Autodesk Inventor part; units mm, degrees
ref_plane "XZ Plane" through (0, 0, 0) normal (0, 1, 0) x (-1, 0, 0)
ref_plane "XY Plane" through (0, 0, 0) normal (0, 0, 1) x (1, 0, 0)
sketch "Sketch1" plane through (0, 0, 0) normal (1, 0, 0) x (0, 1, 0)
  line L0 (0, 67.4997) -> (0, -67.4997)
  line L1 (0, 60) -> (8, 60)
  line L2 (8, 60) -> (8, 42)
  line L3 (8, 42) -> (6, 42)
  line L4 (6, 42) -> (6, 34)
  line L5 (6, 34) -> (12, 34)
  line L6 (12, 34) -> (12, 0)
  line L7 (12, 0) -> (0, 0)
  dimension "d0" = 24
  dimension "d1" = 60
  dimension "d2" = 18
  dimension "d3" = 16
  dimension "d4" = 12
  dimension "d5" = 26
revolve "Revolution1" add sketch "Sketch1" angle 360 about axis through (0, 0, 67.4997) along (0, 0, -1)
chamfer "Chamfer1" distance 1 angle 45 1 edges at (0, -8, 60)
chamfer "Chamfer2" distance 2 angle 45 1 edges at (0, -12, 0)
fillet "Fillet1" radius 2 2 edges at (0, -6, 42) (0, -6, 34)
sketch "Sketch2" plane through (0, 0, 60) normal (0, 0, 1) x (1, 0, 0)
  circle A0 centre (0, 0) radius 7
  point P0 (0, 0)
hole "Hole1" at (0, 0, 60) direction (0, 0, -1) diameter 8.376 depth 22 tip angle 118
sketch "Sketch3" plane through (0, 0, 0) normal (1, 0, 0) x (0, 1, 0)
  line L0 (10, 0) -> (-10, 0)
  line L1 (5, 0) -> (5, 20)
  arc A0 (5, 20) -> (-5, 20) centre (0, 20) ccw
  line L2 (-5, 20) -> (-5, 0)
  line L3 (-5, 0) -> (5, 0)
  point P0 (0, 0)
  dimension "d21" = 10
  dimension "d22" = 20
extrude "Extrusion1" cut sketch "Sketch3" along normal through all both and the other way through all
hole "Hole3" at (0, 12, 10) direction (0, -1, 0) diameter 8.376 end through all
ref_plane "Work Plane2" through (0, 0, 10) normal (0, 0, -1) x (-1, 0, 0)
equation "\"d38\" = 0.5 * d5"
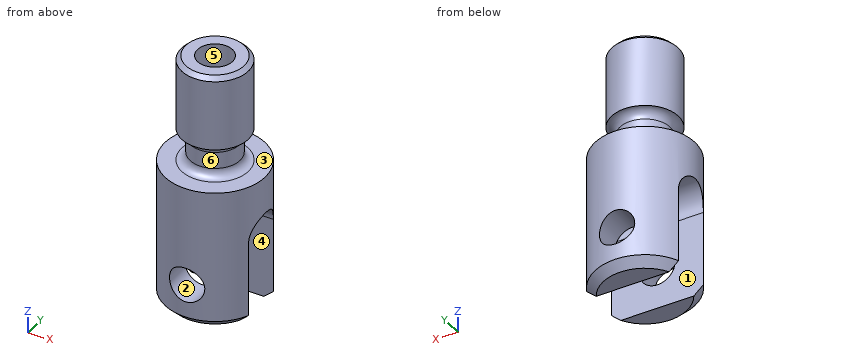
Can you work these out from the model? Positions are in its coordinate system, mm. Face numbers are marked on the shaded views. A direction names the side the tool comes from. Coordinates: 2 decimals unless noted, no trailing zeros. Loops run counter-clockwise (first coordinate to the right, second up) from the corner with the lowest first, then second, coordinate; pieces in that order, holes last.
1) Imagine slicing it at B-B on z = 19. List the corners of the cut face in (x, y) for me.
2) Thinking about a two-plate mould opening in X: for the marked faces 4, 5 and 6, which applies, pulls with the +X half, pulls with the -X half, needs draft (parallel to the pull), parting line crosses it, or undercut?
3) Imagine slicing it at A-A on z = 10. List the corners of the cut face in (x, y) for me, plus the area to 3 significant figures.
4) For pin 1 (8 mm diameter, centred on x = -2.5, y = 0.5, fed in from -Z); pin 2 (10 mm diameter, centred on y = 6, z = 35, fed in from +X); pin 3 (1.5 mm diameter, centred on x = -6, y = 6.5, fed in from +Z), each with a flat end and sliding along its axis, tell me the tip position at first contact or that it passes through.
5) Which directions (+Z, -Z, +X, -X, +Y, -Y) give clear straight access to the entire face, cutting with the end or side of a thin tool? Please do the marked faces 1, 2 and 3.
6) Imagine slicing it at C-C on z = 30.5. List the corners of the cut face in (x, y) for me.
7) I need wall thicknesses on probe 1 along Z at (x, y) = (-0.25, -9.75); probe 2 along X at (y, z) = (0, 54); probe 3 along X at (y, z) = (9.75, 10). Which ranges of each line are inside material? Lowest first, please.
Completed:
1. outline: (-10.91, -5) arc R12 ccw to (10.91, -5) - close; (-10.91, 5) - (10.91, 5) arc R12 ccw to start
2. face 4: needs draft
2. face 5: undercut
2. face 6: parting line crosses it
3. outline: (-10.91, -5) arc R12 ccw to (-4.19, -11.25) - (-4.19, -5) - close; (-10.91, 5) - (-4.19, 5) - (-4.19, 11.25) arc R12 ccw to start; (4.19, -11.25) arc R12 ccw to (10.91, -5) - (4.19, -5) - close; (4.19, 5) - (10.91, 5) arc R12 ccw to (4.19, 11.25) - close
3. area: 106 mm2
4. pin 1: stops at z = 22.18
4. pin 2: stops at x = 11.95
4. pin 3: stops at z = 34
5. face 1: -Z, +X, -X
5. face 2: +Y, -Y
5. face 3: +Z
6. outline: circle Ø24 at (0, 0)
7. probe 1: z = 0 to 5.82, 14.18 to 34
7. probe 2: x = -8 to -4.19, 4.19 to 8
7. probe 3: x = -7 to -4.19, 4.19 to 7
